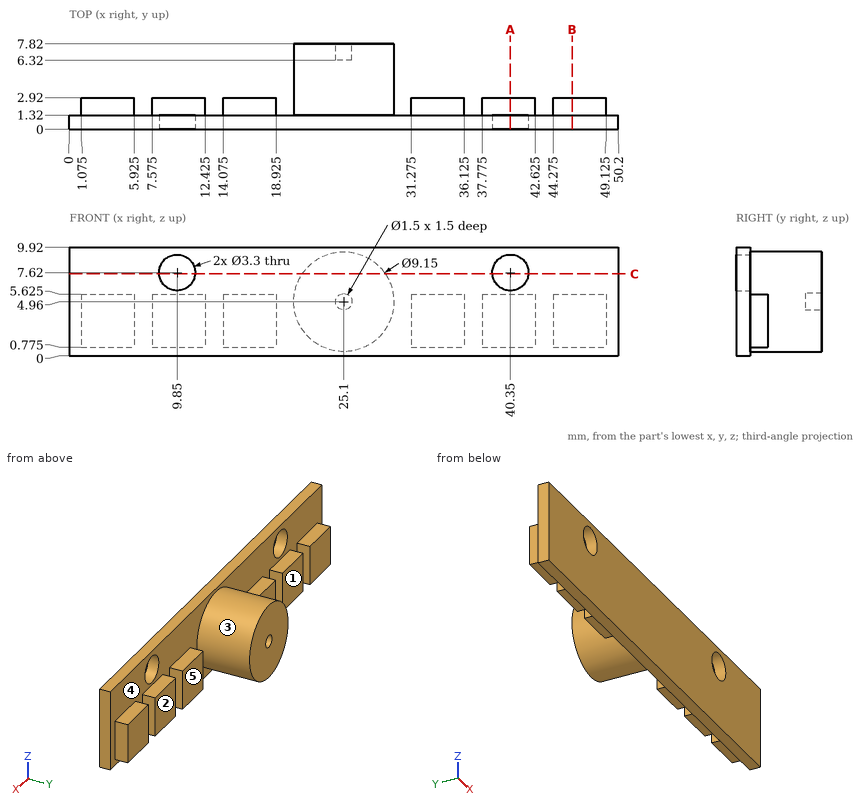
Study the drawing (mm; zero at the part's minimum x, y, z) and answer. A direction names the side the tool comes from. Coordinates: 2 decimals unless noted, no trailing zeros. Order: outer loops, then holes, each group sorted by start corner. A loop starts at its lowest first (then second) coordinate and runs counter-clockwise, first axis right, second up. Notation, with made-up numbers: M 72,85.25 L 116,85.25 A13 ccw 116,89.25 Z; hole C 15,19.5 d11. An arc over 180 degrees is marked long. Answer as a JSON object with one key per item and string values. Group by question number.
1. Determine the mould class of the marked faces 4 and 5 for opening direction X: released by +X, released by -X, zero draft, split by the parting line, or undercut.
2. Flat-ended cylindrical pins translate along their axes: P1, Ø0.8, axis at x = 17, y = 2, coming from the -Z side (3 decimals); P2, Ø1.3, axis at y = 2.5, z = 3, coming from the +X side (3 decimals); P3, Ø1, axis at y = 2.5, z = 8, coming from the +X side; P4, Ø2, axis at x = 44.5, y = 5, coming from the -Z side. Find the tip coordinate at first contact, or state that the pin passes through.
3. Straight lines are drawn through the part: line 1 (X direction, y = 0.55, z = 7.62); line 2 (X direction, y = 7.2, z = 4.96) (3 decimals); line 3 (Y direction, x = 10, z = 3.25). For each, find the intervals that lie inside material, in ascending order.
4. Section C-C on z = 7.5 is taken. Write down the section's boundary in (x, y).
5. A tool of negligible diameter and unlimited length cuts with its end or side. For the marked faces 1, 2 and 3, from which of +Z, -Z, +X, -X, +Y, -Y can it reach the whole face along a straight path? Write none if from no direction.
6. Section B-B on x = 46 is taken. Write down the section's boundary in (y, z) (3 decimals).
7. Section A-A on x = 40.35 is taken. Write down the section's boundary in (y, z) (3 decimals).
Values follow:
{
 "1": {"face 4": "undercut", "face 5": "zero draft"},
 "2": {"P1": "z = 0.775", "P2": "x = 49.125", "P3": "x = 28.91", "P4": "through"},
 "3": {"line 1": "0 to 8.2, 11.5 to 38.7, 42 to 50.2", "line 2": "20.525 to 24.35, 25.85 to 29.675", "line 3": "0 to 2.92"},
 "4": {"outline": "M 0,0 L 8.2,0 L 8.2,1.32 L 0,1.32 Z; M 11.5,0 L 38.7,0 L 38.7,1.32 L 28.91,1.32 L 28.91,7.82 L 21.29,7.82 L 21.29,1.32 L 11.5,1.32 Z; M 42,0 L 50.2,0 L 50.2,1.32 L 42,1.32 Z"},
 "5": {"face 1": "+Z, -Z, -X, +Y", "face 2": "+Z, -Z, +X, +Y", "face 3": "+Y"},
 "6": {"outline": "M 0,0 L 1.32,0 L 1.32,0.775 L 2.92,0.775 L 2.92,5.625 L 1.32,5.625 L 1.32,9.92 L 0,9.92 Z"},
 "7": {"outline": "M 0,0 L 1.32,0 L 1.32,0.775 L 2.92,0.775 L 2.92,5.625 L 1.32,5.625 L 1.32,5.97 L 0,5.97 Z; M 0,9.27 L 1.32,9.27 L 1.32,9.92 L 0,9.92 Z"}
}
